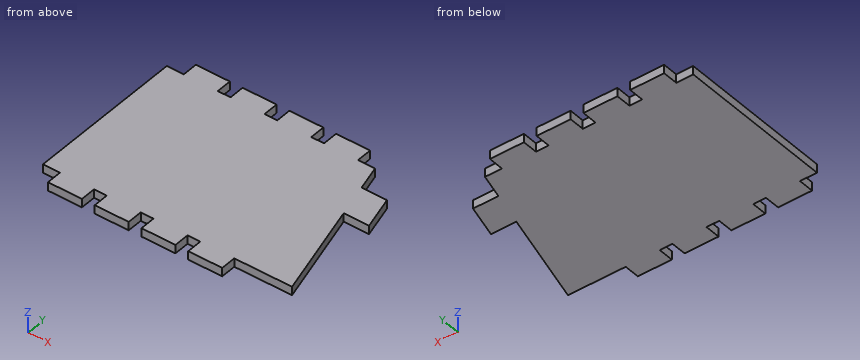
Autodesk Inventor part; units mm, degrees
ref_plane "YZ Plane" through (0, 0, 0) normal (1, 0, 0) x (0, 1, 0)
ref_plane "XZ Plane" through (0, 0, 0) normal (0, 1, 0) x (-1, 0, 0)
ref_plane "XY Plane" through (0, 0, 0) normal (0, 0, 1) x (1, 0, 0)
sketch "Sketch1" plane through (0, 0, 0) normal (0, 0, 1) x (1, 0, 0)
  line L0 (-2.037, -23.495) -> (-2.037, -28.067)
  line L1 (-2.037, -28.067) -> (-12.197, -28.067)
  line L2 (-12.197, -28.067) -> (-12.197, -23.495)
  line L3 (-12.197, -23.495) -> (-16.007, -23.495)
  line L4 (-16.007, -23.495) -> (-16.007, -28.067)
  line L5 (-16.007, -28.067) -> (-26.167, -28.067)
  line L6 (-26.167, -28.067) -> (-26.167, -23.495)
  line L7 (-26.167, -23.495) -> (-29.977, -23.495)
  line L8 (-29.977, -23.495) -> (-29.977, -28.067)
  line L9 (-29.977, -28.067) -> (-40.137, -28.067)
  line L10 (-40.137, -28.067) -> (-40.137, -23.495)
  line L11 (-40.137, -23.495) -> (-43.947, -23.495)
  line L12 (-43.947, -23.495) -> (-43.947, -28.067)
  line L13 (-43.947, -28.067) -> (-54.107, -28.067)
  line L14 (-54.107, -28.067) -> (-54.107, -23.495)
  line L15 (-54.107, -23.495) -> (-59.187, -23.495)
  line L16 (3.043, 23.495) -> (-2.037, 23.495)
  line L17 (-2.037, 23.495) -> (-2.037, 28.067)
  line L18 (-2.037, 28.067) -> (-12.197, 28.067)
  line L19 (-12.197, 28.067) -> (-12.197, 23.495)
  line L20 (-12.197, 23.495) -> (-16.007, 23.495)
  line L21 (-16.007, 23.495) -> (-16.007, 28.067)
  line L22 (-16.007, 28.067) -> (-26.167, 28.067)
  line L23 (-26.167, 28.067) -> (-26.167, 23.495)
  line L24 (-26.167, 23.495) -> (-29.977, 23.495)
  line L25 (-29.977, 23.495) -> (-29.977, 28.067)
  line L26 (-29.977, 28.067) -> (-40.137, 28.067)
  line L27 (-40.137, 28.067) -> (-40.137, 23.495)
  line L28 (-40.137, 23.495) -> (-43.947, 23.495)
  line L29 (-43.947, 23.495) -> (-43.947, 28.067)
  line L30 (-43.947, 28.067) -> (-54.107, 28.067)
  line L31 (-54.107, 28.067) -> (-54.107, 23.495)
  line L32 (-54.107, 23.495) -> (-59.187, 23.495)
  line L33 (-59.187, 23.495) -> (-59.187, -23.495)
  line L34 (15.235, 5.7718) -> (15.235, 5.715)
  line L35 (15.235, 5.715) -> (7.6562, 5.715)
  line L36 (12.6136, 15.875) -> (15.235, 5.7718)
  line L37 (3.043, 23.495) -> (5.0201, 15.875)
  line L38 (7.6562, 5.715) -> (15.235, -23.495)
  line L39 (5.0201, 15.875) -> (12.6136, 15.875)
  line L40 (-2.037, -23.495) -> (15.235, -23.495)
  dimension "d11" = 4.572
  dimension "d12" = 10.16
  dimension "d13" = 3.81
  dimension "d14" = 10.16
  dimension "d15" = 3.81
  dimension "d16" = 10.16
  dimension "d17" = 3.81
  dimension "d18" = 10.16
  dimension "d19" = 5.08
  dimension "d34" = 4.572
  dimension "d84" = 7.62
  dimension "d85" = 29.21
  dimension "d86" = 10.1032
extrude "Extrusion4" add sketch "Sketch1" along normal blind 2.54
properties part number "RTS Frame Sides"
Could you check a few things on this model? Use its own coordinates, in mm. Give positions to 0.01 mm unless a question says otherwise; leave off trailing zeros. Order: outer loops, then holes, each group sorted by start corner. A loop starts at its lowest first (then second) coordinate and runs counter-clockwise, first axis right, second up. Notation, with made-up numbers: (-21, 16) - (29, 16) arc R19 cw to (29, 50) - close; hole circle Ø9 at (-5, 17). An arc over 180 degrees is marked (long way). Return JSON: item names as keys, results as strings. Group by question number.
Q1. Please list where these lines run through material, in increasing order: line 1 along X through (y, z) = (-25, 1.2); line 2 along Y through (x, z) = (-27.5, 1.45) (3 decimals); line 3 along X through (y, z) = (7, 0.25). Write a range as [from, to].
Q2. Suppose I cut it at C-C, the plane y = -3. Please give me the cut outline in (x, z), and give its area (3 significant figures).
Q3. Suppose I cut it at A-A, the plane y = 24.5. Please give me the cut outline in (x, z), and give its area (3 significant figures).
Q4. Suppose I cut it at B-B, the plane x = -13. Please give me the cut outline in (y, z) (3 decimals).
Q5. Will these pins go through, and if not, where does the flat tip stop? pin 1 Ø1.3 at (y, z) = (25, 1.5) entering from -X; pin 2 Ø1.3 at (x, z) = (12.5, 1.5) entering from -Y (3 decimals); pin 3 Ø0.8 at (x, z) = (-55.5, 1) entering from +Y (3 decimals).
Resolved:
{
 "1": {"line 1": "x = [-54.11, -43.95], [-40.14, -29.98], [-26.17, -16.01], [-12.2, -2.04]", "line 2": "y = [-23.495, 23.495]", "line 3": "x = [-59.19, 14.92]"},
 "2": {"outline": "(-59.19, 0) - (9.92, 0) - (9.92, 2.54) - (-59.19, 2.54) - close", "area": "176 mm2"},
 "3": {"outline": "(-54.11, 0) - (-43.95, 0) - (-43.95, 2.54) - (-54.11, 2.54) - close; (-40.14, 0) - (-29.98, 0) - (-29.98, 2.54) - (-40.14, 2.54) - close; (-26.17, 0) - (-16.01, 0) - (-16.01, 2.54) - (-26.17, 2.54) - close; (-12.2, 0) - (-2.04, 0) - (-2.04, 2.54) - (-12.2, 2.54) - close", "area": "103 mm2"},
 "4": {"outline": "(-23.495, 0) - (23.495, 0) - (23.495, 2.54) - (-23.495, 2.54) - close"},
 "5": {"pin 1": "stops at x = -54.11", "pin 2": "stops at y = -23.495", "pin 3": "stops at y = 23.495"}
}
